Can you work these out from the model? Positions are in its coordinate system, mm. A direction names the side the tool comes from. Round coordinates to 2 decimals unless told otherwise and drop trailing zeros.
Q1. I'm going to push flat-ended pins straight in: pin 1 Ø1.1 at (x, y) = (0, 23.5) entering from -Z; pin 2 Ø1 at (x, y) = (18, 35) entering from -Z; pin 3 Ø0.5 at (x, z) = (-10, 0) entering from -Y. Where does each tip first touch, or does it pass through?
Q2. Please list where these lines run through material, in increasing order: line 1 along X through (y, z) = (5.25, 0) (3 decimals); line 2 along Z through (x, y) = (-12, 29); line 3 along Z through (x, y) = (11, 17.5).
Q3. We'd pull the mould along Z, two halves only. Please class faces 1 (the flat face through (1.134, 34.51, -23.49)), 2 (the flat face through (9.51, 34.51, 21.46)), 3 (the flat face through (-22.283, 34.51, -7.519)): +Z half, -Z half, draft (parallel to the pull), parting line (faces both ways), or undercut.
Q4. For faces 4 (the flat face through (-13.293, 34.51, -19.349)), 5 (the flat face through (23.246, 34.51, -3.275)), 6 (the cylindrical face through (-3.905, 4.93, 0.867)), 7 (the flat face through (19.43, 34.51, -13.25)), 8 (the flat face through (-23.452, 34.51, -1.052)), which set-ups out of +Z, -Z, +X, -X, +Y, -Y let a thin tool reach every point of the face, with its end or its side?
Q5. If we section it at A-A (y = 38.5): Give the number of separate pieces and of enclosed holes in the cut face, plus the area to 3 significant figures.
from build123d import *

# Parameters (mm, degrees)
BOSS_EXTRUDE2_DEPTH = 70
SKETCH3_R           = 4
CUT_EXTRUDE1_DEPTH  = 10
SKETCH4_R           = 0.5
CUT_EXTRUDE2_DEPTH  = 10
CIRPATTERN1_COUNT   = 2
CUT_EXTRUDE3_DEPTH  = 79.402407488


# Read off the part's stored shape, not the designer's step: Boss-Extrude2
with BuildPart() as part:
    # Boss-Extrude2 outline → Boss-Extrude2 (new body)
    with BuildSketch(Plane(origin=(0, 0, 0), x_dir=(1, 0, 0), z_dir=(0, 1, 0))):
        with BuildLine():
            Line((1.75, 24.938674784), (0.5, 22))
            Line((0.5, 22), (-0.5, 22))
            Line((-0.5, 22), (-1.75, 24.938674784))
            ThreePointArc((-1.75, 24.938674784), (-2.306708986, 24.893354407), (-2.862266542, 24.835608111))
            Line((-2.862266542, 24.835608111), (-3.551002842, 21.717282952))
            Line((-3.551002842, 21.717282952), (-4.533975942, 21.533533434))
            Line((-4.533975942, 21.533533434), (-6.302672391, 24.192484799))
            ThreePointArc((-6.302672391, 24.192484799), (-6.841574752, 24.045641079), (-7.37706203, 23.88679459))
            Line((-7.37706203, 23.88679459), (-7.481080541, 20.69500988))
            Line((-7.481080541, 20.69500988), (-8.413552771, 20.333768214))
            Line((-8.413552771, 20.333768214), (-10.640714833, 22.622448759))
            ThreePointArc((-10.640714833, 22.622448759), (-11.143458894, 22.379082284), (-11.640640518, 22.124544929))
            Line((-11.640640518, 22.124544929), (-11.156399015, 18.967993067))
            Line((-11.156399015, 18.967993067), (-12.006616151, 18.441560905))
            Line((-12.006616151, 18.441560905), (-14.616400494, 20.282032359))
            ThreePointArc((-14.616400494, 20.282032359), (-15.065865909, 19.950430682), (-15.507810955, 19.608870426))
            Line((-15.507810955, 19.608870426), (-14.451799702, 16.595044001))
            Line((-14.451799702, 16.595044001), (-15.190808619, 15.921348357))
            Line((-15.190808619, 15.921348357), (-18.094342166, 17.250935673))
            ThreePointArc((-18.094342166, 17.250935673), (-18.475222931, 16.842391091), (-18.84688149, 16.425439358))
            Line((-18.84688149, 16.425439358), (-17.255061682, 13.656970614))
            Line((-17.255061682, 13.656970614), (-17.857696318, 12.858953387))
            Line((-17.857696318, 12.858953387), (-20.956102717, 13.632379063))
            ThreePointArc((-20.956102717, 13.632379063), (-21.255428393, 13.160804072), (-21.544144079, 12.682659653))
            Line((-21.544144079, 12.682659653), (-19.470723232, 10.253825473))
            Line((-19.470723232, 10.253825473), (-19.916461588, 9.358662181))
            Line((-19.916461588, 9.358662181), (-23.104228325, 9.549588134))
            ThreePointArc((-23.104228325, 9.549588134), (-23.311805735, 9.031041654), (-23.507746682, 8.507987185))
            Line((-23.507746682, 8.507987185), (-21.023332655, 6.501498603))
            Line((-21.023332655, 6.501498603), (-21.296995645, 5.53967296))
            Line((-21.296995645, 5.53967296), (-24.465567147, 5.141597434))
            ThreePointArc((-24.465567147, 5.141597434), (-24.574327492, 4.593737945), (-24.670821165, 4.043585418))
            Line((-24.670821165, 4.043585418), (-21.860017699, 2.527770996))
            Line((-21.860017699, 2.527770996), (-21.952286058, 1.53203682))
            Line((-21.952286058, 1.53203682), (-24.993760423, 0.558515801))
            ThreePointArc((-24.993760423, 0.558515801), (-25, 0), (-24.993760423, -0.558515801))
            Line((-24.993760423, -0.558515801), (-21.952286058, -1.53203682))
            Line((-21.952286058, -1.53203682), (-21.860017699, -2.527770996))
            Line((-21.860017699, -2.527770996), (-24.670821165, -4.043585418))
            ThreePointArc((-24.670821165, -4.043585418), (-24.574327492, -4.593737945), (-24.465567147, -5.141597434))
            Line((-24.465567147, -5.141597434), (-21.296995645, -5.53967296))
            Line((-21.296995645, -5.53967296), (-21.023332655, -6.501498603))
            Line((-21.023332655, -6.501498603), (-23.507746682, -8.507987185))
            ThreePointArc((-23.507746682, -8.507987185), (-23.311805735, -9.031041654), (-23.104228325, -9.549588134))
            Line((-23.104228325, -9.549588134), (-19.916461588, -9.358662181))
            Line((-19.916461588, -9.358662181), (-19.470723232, -10.253825473))
            Line((-19.470723232, -10.253825473), (-21.544144079, -12.682659654))
            ThreePointArc((-21.544144079, -12.682659654), (-21.255428393, -13.160804072), (-20.956102717, -13.632379063))
            Line((-20.956102717, -13.632379063), (-17.857696318, -12.858953387))
            Line((-17.857696318, -12.858953387), (-17.255061682, -13.656970614))
            Line((-17.255061682, -13.656970614), (-18.84688149, -16.425439358))
            ThreePointArc((-18.84688149, -16.425439358), (-18.475222931, -16.842391091), (-18.094342166, -17.250935673))
            Line((-18.094342166, -17.250935673), (-15.190808619, -15.921348357))
            Line((-15.190808619, -15.921348357), (-14.451799702, -16.595044001))
            Line((-14.451799702, -16.595044001), (-15.507810955, -19.608870426))
            ThreePointArc((-15.507810955, -19.608870426), (-15.065865909, -19.950430682), (-14.616400494, -20.282032359))
            Line((-14.616400494, -20.282032359), (-12.006616151, -18.441560905))
            Line((-12.006616151, -18.441560905), (-11.156399015, -18.967993067))
            Line((-11.156399015, -18.967993067), (-11.640640518, -22.124544929))
            ThreePointArc((-11.640640518, -22.124544929), (-11.143458894, -22.379082284), (-10.640714833, -22.622448759))
            Line((-10.640714833, -22.622448759), (-8.413552771, -20.333768214))
            Line((-8.413552771, -20.333768214), (-7.481080541, -20.69500988))
            Line((-7.481080541, -20.69500988), (-7.37706203, -23.88679459))
            ThreePointArc((-7.37706203, -23.88679459), (-6.841574752, -24.045641079), (-6.302672391, -24.192484799))
            Line((-6.302672391, -24.192484799), (-4.533975942, -21.533533434))
            Line((-4.533975942, -21.533533434), (-3.551002842, -21.717282952))
            Line((-3.551002842, -21.717282952), (-2.862266542, -24.835608111))
            ThreePointArc((-2.862266542, -24.835608111), (-2.306708986, -24.893354407), (-1.75, -24.938674784))
            Line((-1.75, -24.938674784), (-0.5, -22))
            Line((-0.5, -22), (0.5, -22))
            Line((0.5, -22), (1.75, -24.938674784))
            ThreePointArc((1.75, -24.938674784), (2.306708986, -24.893354407), (2.862266542, -24.835608111))
            Line((2.862266542, -24.835608111), (3.551002842, -21.717282952))
            Line((3.551002842, -21.717282952), (4.533975942, -21.533533434))
            Line((4.533975942, -21.533533434), (6.302672391, -24.192484799))
            ThreePointArc((6.302672391, -24.192484799), (6.841574752, -24.045641079), (7.37706203, -23.88679459))
            Line((7.37706203, -23.88679459), (7.481080541, -20.69500988))
            Line((7.481080541, -20.69500988), (8.413552771, -20.333768214))
            Line((8.413552771, -20.333768214), (10.640714833, -22.622448759))
            ThreePointArc((10.640714833, -22.622448759), (11.143458895, -22.379082284), (11.640640519, -22.124544929))
            Line((11.640640519, -22.124544929), (11.156399015, -18.967993067))
            Line((11.156399015, -18.967993067), (12.006616151, -18.441560905))
            Line((12.006616151, -18.441560905), (14.616400494, -20.282032359))
            ThreePointArc((14.616400494, -20.282032359), (15.065865909, -19.950430682), (15.507810955, -19.608870426))
            Line((15.507810955, -19.608870426), (14.451799702, -16.595044001))
            Line((14.451799702, -16.595044001), (15.190808619, -15.921348357))
            Line((15.190808619, -15.921348357), (18.094342166, -17.250935673))
            ThreePointArc((18.094342166, -17.250935673), (18.475222931, -16.842391091), (18.84688149, -16.425439358))
            Line((18.84688149, -16.425439358), (17.255061682, -13.656970614))
            Line((17.255061682, -13.656970614), (17.857696318, -12.858953387))
            Line((17.857696318, -12.858953387), (20.956102717, -13.632379063))
            ThreePointArc((20.956102717, -13.632379063), (21.255428393, -13.160804072), (21.544144079, -12.682659653))
            Line((21.544144079, -12.682659653), (19.470723232, -10.253825473))
            Line((19.470723232, -10.253825473), (19.916461588, -9.358662181))
            Line((19.916461588, -9.358662181), (23.104228325, -9.549588134))
            ThreePointArc((23.104228325, -9.549588134), (23.311805735, -9.031041654), (23.507746682, -8.507987185))
            Line((23.507746682, -8.507987185), (21.023332655, -6.501498603))
            Line((21.023332655, -6.501498603), (21.296995645, -5.53967296))
            Line((21.296995645, -5.53967296), (24.465567147, -5.141597434))
            ThreePointArc((24.465567147, -5.141597434), (24.574327492, -4.593737945), (24.670821165, -4.043585418))
            Line((24.670821165, -4.043585418), (21.860017699, -2.527770996))
            Line((21.860017699, -2.527770996), (21.952286058, -1.53203682))
            Line((21.952286058, -1.53203682), (24.993760423, -0.558515801))
            ThreePointArc((24.993760423, -0.558515801), (25, 0), (24.993760423, 0.558515801))
            Line((24.993760423, 0.558515801), (21.952286058, 1.53203682))
            Line((21.952286058, 1.53203682), (21.860017699, 2.527770996))
            Line((21.860017699, 2.527770996), (24.670821165, 4.043585418))
            ThreePointArc((24.670821165, 4.043585418), (24.574327492, 4.593737945), (24.465567147, 5.141597434))
            Line((24.465567147, 5.141597434), (21.296995645, 5.53967296))
            Line((21.296995645, 5.53967296), (21.023332655, 6.501498603))
            Line((21.023332655, 6.501498603), (23.507746682, 8.507987185))
            ThreePointArc((23.507746682, 8.507987185), (23.311805735, 9.031041654), (23.104228325, 9.549588134))
            Line((23.104228325, 9.549588134), (19.916461588, 9.358662181))
            Line((19.916461588, 9.358662181), (19.470723232, 10.253825473))
            Line((19.470723232, 10.253825473), (21.544144079, 12.682659653))
            ThreePointArc((21.544144079, 12.682659653), (21.255428393, 13.160804072), (20.956102717, 13.632379063))
            Line((20.956102717, 13.632379063), (17.857696318, 12.858953387))
            Line((17.857696318, 12.858953387), (17.255061682, 13.656970614))
            Line((17.255061682, 13.656970614), (18.84688149, 16.425439358))
            ThreePointArc((18.84688149, 16.425439358), (18.475222931, 16.842391091), (18.094342166, 17.250935673))
            Line((18.094342166, 17.250935673), (15.190808619, 15.921348357))
            Line((15.190808619, 15.921348357), (14.451799702, 16.595044001))
            Line((14.451799702, 16.595044001), (15.507810955, 19.608870426))
            ThreePointArc((15.507810955, 19.608870426), (15.065865909, 19.950430682), (14.616400494, 20.282032359))
            Line((14.616400494, 20.282032359), (12.006616151, 18.441560905))
            Line((12.006616151, 18.441560905), (11.156399015, 18.967993067))
            Line((11.156399015, 18.967993067), (11.640640518, 22.124544929))
            ThreePointArc((11.640640518, 22.124544929), (11.143458894, 22.379082284), (10.640714833, 22.622448759))
            Line((10.640714833, 22.622448759), (8.413552771, 20.333768214))
            Line((8.413552771, 20.333768214), (7.481080541, 20.69500988))
            Line((7.481080541, 20.69500988), (7.37706203, 23.88679459))
            ThreePointArc((7.37706203, 23.88679459), (6.841574752, 24.045641079), (6.302672391, 24.192484799))
            Line((6.302672391, 24.192484799), (4.533975942, 21.533533434))
            Line((4.533975942, 21.533533434), (3.551002842, 21.717282952))
            Line((3.551002842, 21.717282952), (2.862266542, 24.835608111))
            ThreePointArc((2.862266542, 24.835608111), (2.306708986, 24.893354407), (1.75, 24.938674784))
        make_face()
    extrude(amount=BOSS_EXTRUDE2_DEPTH)

    # Sketch3 → Cut-Extrude1 (cut)
    with BuildSketch(Plane.XZ):
        with Locations(Location((0, 0, 0), (0, 0, 270))):
            Circle(SKETCH3_R)
    extrude(amount=-CUT_EXTRUDE1_DEPTH, mode=Mode.SUBTRACT)

    # Sketch4 → Cut-Extrude2 (cut)
    with BuildSketch(Plane.XZ):
        with Locations(Location((-9.925, 0, 0), (0, 0, 270))):
            Circle(SKETCH4_R)
    cut_extrude2 = extrude(amount=-CUT_EXTRUDE2_DEPTH, mode=Mode.SUBTRACT)

    # CirPattern1: Cut-Extrude2 ×2 about axis
    cirpattern1_axis = Axis((0, 0, 0), (0, 1, 0))
    for i in range(1, CIRPATTERN1_COUNT):
        add(cut_extrude2.rotate(cirpattern1_axis, i * 360 / CIRPATTERN1_COUNT), mode=Mode.SUBTRACT)

    # Sketch5 → Cut-Extrude3 (cut, through all)
    with BuildSketch(Plane.XZ):
        with BuildLine():
            Line((-12.5, 6.623664739), (12.5, 6.623664739))
            ThreePointArc((12.5, 6.623664739), (0, 15.524722913), (-12.5, 6.623664739))
        make_face()
        with BuildLine():
            Line((12.5, -6.623664739), (-12.5, -6.623664739))
            ThreePointArc((-12.5, -6.623664739), (0, -15.524722913), (12.5, -6.623664739))
        make_face()
    extrude(amount=-CUT_EXTRUDE3_DEPTH, mode=Mode.SUBTRACT)


solid = part.part
A:
1. pin 1: stops at z = -22.12
1. pin 2: stops at z = -17.25
1. pin 3: stops at y = 10
2. line 1: x = -25 to -10.425, -9.425 to -4, 4 to 9.425, 10.425 to 25
2. line 2: z = -18.45 to -7.86, -6.62 to 6.62, 7.86 to 18.45
2. line 3: z = -22.45 to -9.64, -6.62 to 6.62, 9.64 to 22.45
3. face 1: -Z half
3. face 2: +Z half
3. face 3: undercut
4. face 4: -Z, +Y, -Y
4. face 5: +X, +Y, -Y
4. face 6: -Y
4. face 7: +Y, -Y
4. face 8: -X, +Y, -Y
5. separate pieces: 1
5. enclosed holes: 2
5. area: 1,410 mm2
